Check sheet for the modelled part. Datum: model origin and axes. Units: mm. Face numbers are marked on the shaded views. A direction names the side the tool comes from. Round coordinates to 2 decimals unless told otherwise and drop trailing zeros. Loops run counter-clockwise (first coordinate to the right, second up) from the corner with the lowest first, then second, coordinate; pieces in that order, holes last. Notation, with made-up numbers: (65, 30) -> (95, 30) arc R19 cw to (95, 44) -> close; hole circle Ø11 at (-8.5, 42.25). An arc over 180 degrees is marked (long way). Return JSON: item names as keys, results as strings.
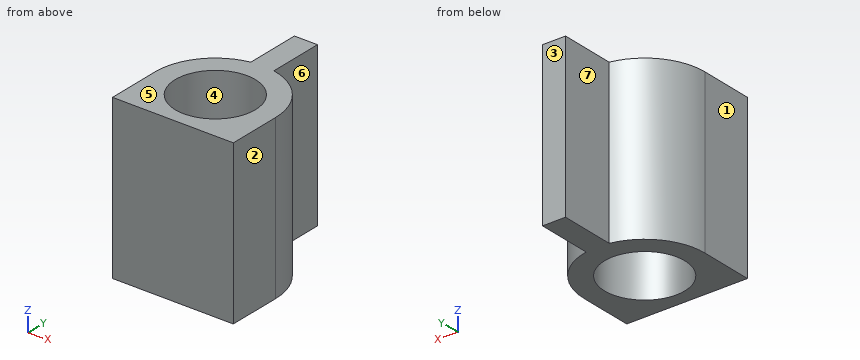
from build123d import *

# Parameters (mm, degrees)
SKETCH1_R           = 11.049
BOSS_EXTRUDE1_DEPTH = 22.225


with BuildPart() as part:
    # Sketch1 → Boss-Extrude1 (new, symmetric)
    with BuildSketch(Plane.XY):
        with BuildLine():
            Line((16.637, -14.732), (-16.637, -14.732))
            Line((-16.637, -14.732), (-16.637, 0))
            ThreePointArc((-16.637, 0), (-12.83768367, 10.582232609), (-3.175, 16.331232164))
            Line((-3.175, 16.331232164), (-3.175, 31.496))
            Line((-3.175, 31.496), (3.175, 31.496))
            Line((3.175, 31.496), (3.175, 16.331232164))
            ThreePointArc((3.175, 16.331232164), (12.83768367, 10.582232609), (16.637, 0))
            Line((16.637, 0), (16.637, -14.732))
        make_face()
        Circle(SKETCH1_R, mode=Mode.SUBTRACT)
    extrude(amount=BOSS_EXTRUDE1_DEPTH, both=True)


solid = part.part
Q1. Section check C-C (z = 3). Record the boundary of the cut face in (x, y) (3 decimals), then the cut area to 3 significant figures.
Results list:
{"outline": "(-16.637, -14.732) -> (16.637, -14.732) -> (16.637, 0) arc R16.637 ccw to (3.175, 16.331) -> (3.175, 31.496) -> (-3.175, 31.496) -> (-3.175, 16.331) arc R16.637 ccw to (-16.637, 0) -> close; hole circle Ø22.098 at (0, 0)", "area": "636 mm^2"}
Q2. Section check A-A (x = 0). Record the boundary of the cut face in (y, z) (3 decimals), then the cut area to 3 significant figures.
Results list:
{"outline": "(-14.732, -22.225) -> (-11.049, -22.225) -> (-11.049, 22.225) -> (-14.732, 22.225) -> close; (11.049, -22.225) -> (31.496, -22.225) -> (31.496, 22.225) -> (11.049, 22.225) -> close", "area": "1,070 mm^2"}
Q3. Material ranges on line 1 (Y direction, x = 0, z = 13); line 2 (X direction, y = 6.5, z = -7); line 3 (Y direction, x = -7, z = -10), recorded low to high.
Results list:
{"line 1": "-14.73 to -11.05, 11.05 to 31.5", "line 2": "-15.31 to -8.93, 8.93 to 15.31", "line 3": "-14.73 to -8.55, 8.55 to 15.09"}
Q4. Draft check along X on the marked faces 1, 2, 3 and 4. Enter one of: released by +X, released by -X, zero draft, split by the parting line, or undercut.
Results list:
{"face 1": "released by -X", "face 2": "released by +X", "face 3": "zero draft", "face 4": "undercut"}
Q5. Tool access check on the marked faces 5, 6 and 7. Record the directions out of +Z, -Z, +X, -X, +Y, -Y that give a thin tool (end or side, any length) a straight path to the whole face; none if there is none.
Results list:
{"face 5": "+Z, +X, -X, +Y, -Y", "face 6": "+Z, -Z, +X, +Y", "face 7": "+Z, -Z, -X, +Y"}
Q6. Section check B-B (y = -3). Record the boundary of the cut face in (x, z) (3 decimals).
Results list:
{"outline": "(-16.637, -22.225) -> (-10.634, -22.225) -> (-10.634, 22.225) -> (-16.637, 22.225) -> close; (10.634, -22.225) -> (16.637, -22.225) -> (16.637, 22.225) -> (10.634, 22.225) -> close"}
Q7. Section check D-D (y = 25.5). Record the boundary of the cut face in (x, z) (3 decimals).
Results list:
{"outline": "(-3.175, -22.225) -> (3.175, -22.225) -> (3.175, 22.225) -> (-3.175, 22.225) -> close"}
Q8. Go/stop test with flat-tipped pins: pin 1 (16.5 mm diameter, centred on y = 27.5, z = 2.5, fed in from +X) (3 decimals); pin 2 (1.5 mm diameter, centred on x = -4.5, z = -11, fed in from +Y); pin 3 (2 mm diameter, centred on x = -8, z = 16, fed in from +Y); pin 4 (10 mm diameter, centred on x = -7, z = 17.5, fed in from +Y). Record where each tip stops, or that it passes through.
Results list:
{"pin 1": "x = 3.175", "pin 2": "y = 16.21", "pin 3": "y = 15.09", "pin 4": "y = 31.5"}
